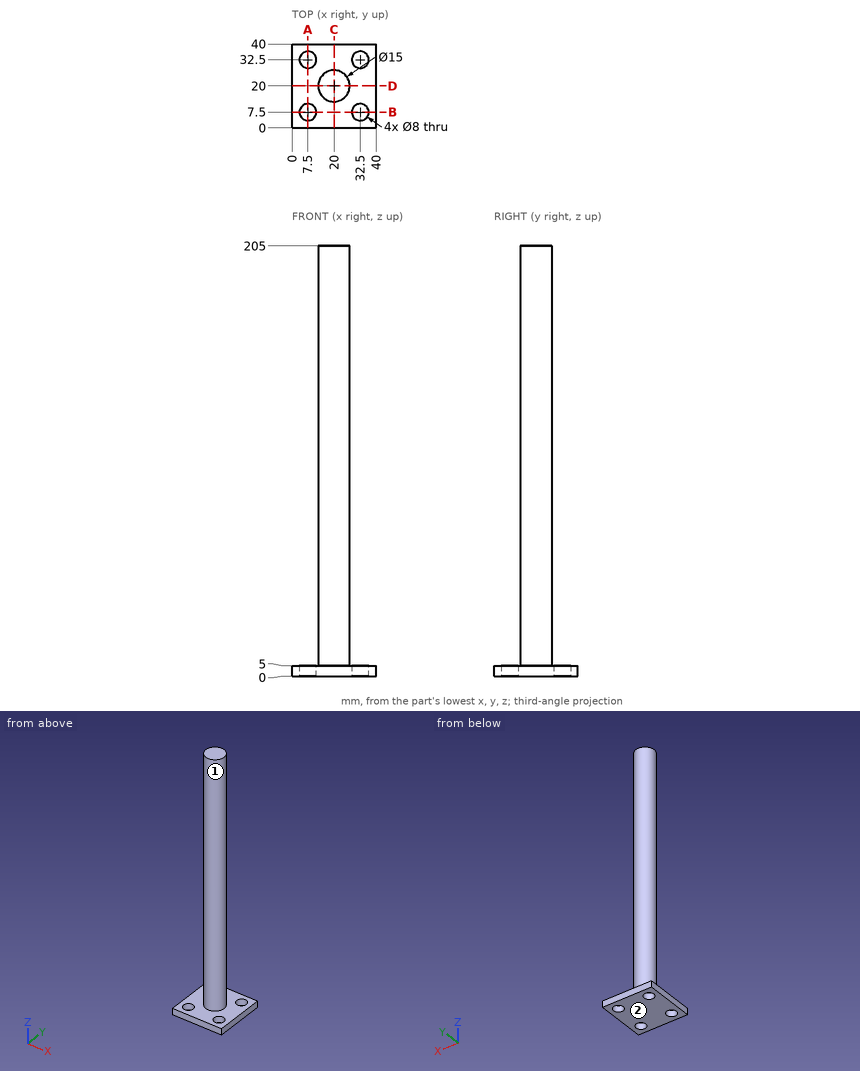
Part print with two shaded views. Sizes in mm from the minimum x, y, z corner. A direction names the side the tool comes from. Round coordinates to 2 decimals unless told otherwise and drop trailing zeros. Write each loop counter-clockwise with the first axis right and the second up, starting at its lowest first coordinate (ties: lowest second). Pieces come first, ordered by that corner, then holes. Notation, with made-up numbers: M 16.5,-22.5 L 58.5,-22.5 A31 cw 58.5,14.5 Z; hole C 14.25,27.25 d6. An arc over 180 degrees is marked long. Put each result on its own line as item: value. Start each with the question number.
1) Saw through at C-C, the plane x = 20. Write the cut outline in (y, z), and give its area (3 significant figures).
2) 3-axis set-ups, long thin cutter, end or side, ignore diameter. For the marked faces 1 and 2: which of +Z, -Z, +X, -X, +Y, -Y reach the whole face in a straight line?
3) Pin check, flat tips, straight feed: pin 1 Ø6.5 at (x, y) = (7.5, 7.5) entering from -Z; pin 2 Ø6 at (x, y) = (17, 32.5) entering from -Z; pin 3 Ø5 at (y, z) = (20, 41.5) entering from +X; pin 4 Ø12 at (x, z) = (32.5, 94.5) entering from +Y. Stop position of each tip, or through.
4) Saw through at A-A, the plane x = 7.5. Write the cut outline in (y, z).
5) Drill centre lines: probe 1 along Y at (x, z) = (7, 3); probe 2 along X at (y, z) = (19.5, 139). Where is each one in solid material? Low to high. Write a range as [from, to].
Resolved:
1. outline: M 0,0 L 40,0 L 40,5 L 27.5,5 L 27.5,205 L 12.5,205 L 12.5,5 L 0,5 Z
1. area: 3,200 mm²
2. face 1: +Z
2. face 2: -Z, +X, -X, +Y, -Y
3. pin 1: through
3. pin 2: z = 0
3. pin 3: x = 27.5
3. pin 4: y = 23.74
4. outline: M 0,0 L 3.5,0 L 3.5,5 L 0,5 Z; M 11.5,0 L 28.5,0 L 28.5,5 L 11.5,5 Z; M 36.5,0 L 40,0 L 40,5 L 36.5,5 Z
5. probe 1: [0, 3.53], [11.47, 28.53], [36.47, 40]
5. probe 2: [12.52, 27.48]
